```python
from build123d import *

# Parameters (mm, degrees)
SKETCH_1_R          = 17
EXTRUDE_1_DEPTH     = 6
SKETCH_2_R          = 7
EXTRUDE_2_DEPTH     = 6
SKETCH_3_R          = 18
EXTRUDE_3_DEPTH     = 5
EXTRUDE_START       = -5
EXTRUDE_6_DEPTH     = 5
CUT_EXTRUDE_1_DEPTH = 8
SKETCH_6_R          = 3.275
EXTRUDE_5_DEPTH     = 4.4
SKETCH_9_R          = 5
CUT_EXTRUDE_3_DEPTH = 37.608729958
SKETCH_10_R         = 13.6
SKETCH_10_R_2       = 8.6
CUT_EXTRUDE_4_DEPTH = 3


with BuildPart() as part:
    # 스케치1 → 보스-돌출1 (new body)
    with BuildSketch(Plane.XY):
        Circle(SKETCH_1_R)
    extrude(amount=EXTRUDE_1_DEPTH)

    # 스케치2 → 보스-돌출2 (add)
    with BuildSketch(Plane.XY.offset(6)):
        Circle(SKETCH_2_R)
    extrude(amount=EXTRUDE_2_DEPTH)

    # 스케치3 → 보스-돌출3 (add)
    with BuildSketch(Plane(origin=(0, 0, 0), x_dir=(-1, 0, 0), z_dir=(0, 0, -1))):
        Circle(SKETCH_3_R)
    extrude(amount=EXTRUDE_3_DEPTH)

    # 스케치8 → 보스-돌출6 (add)
    with BuildSketch(Plane(origin=(0, 0, -5), x_dir=(-1, 0, 0), z_dir=(0, 0, -1)).offset(EXTRUDE_START)):
        with BuildLine():
            Line((-10, 14.966629547), (-10, 26.966629547))
            Line((-10, 26.966629547), (10, 26.966629547))
            Line((10, 26.966629547), (10, 14.966629547))
            ThreePointArc((10, 14.966629547), (0, 18), (-10, 14.966629547))
        make_face()
    extrude_6 = extrude(amount=EXTRUDE_6_DEPTH)

    # 스케치5 → 컷-돌출1 (cut)
    with BuildSketch(Plane.XY):
        Polygon((-10, 27), (-10, 15), (-4, 27), align=None)
        Polygon((4, 27), (10, 27), (10, 15), align=None)
    cut_extrude_1 = extrude(amount=-CUT_EXTRUDE_1_DEPTH, mode=Mode.SUBTRACT)

    # 스케치6 → 보스-돌출5 (add)
    with BuildSketch(Plane.XY):
        with Locations(Location((0, 21.966629547, 0), (0, 0, 180))):
            Circle(SKETCH_6_R)
    extrude_5 = extrude(amount=EXTRUDE_5_DEPTH)

    # 대칭 복사6: 보스-돌출6, 컷-돌출1, 보스-돌출5 across plane
    add(extrude_6.mirror(Plane.ZX))
    add(cut_extrude_1.mirror(Plane.ZX), mode=Mode.SUBTRACT)
    add(extrude_5.mirror(Plane.ZX))

    # 스케치9 → 컷-돌출3 (cut, through all)
    with BuildSketch(Plane.XY.offset(12)):
        Circle(SKETCH_9_R)
    extrude(amount=-CUT_EXTRUDE_3_DEPTH, mode=Mode.SUBTRACT)

    # 스케치10 → 컷-돌출4 (cut)
    with BuildSketch(Plane(origin=(0, 0, -5), x_dir=(-1, 0, 0), z_dir=(0, 0, -1))):
        Circle(SKETCH_10_R)
        Circle(SKETCH_10_R_2, mode=Mode.SUBTRACT)
    extrude(amount=-CUT_EXTRUDE_4_DEPTH, mode=Mode.SUBTRACT)


solid = part.part
```
The model under review builds one solid part; all positions refer to its coordinate system, in mm. A direction names the side the tool comes from. Round coordinates to 2 decimals unless told otherwise and drop trailing zeros. Loops run counter-clockwise (first coordinate to the right, second up) from the corner with the lowest first, then second, coordinate; pieces in that order, holes last. Notation, with made-up numbers: (18, 73) -> (60, 73) arc R34 ccw to (60, 108) -> close; hole circle Ø5 at (39, 84). An arc over 180 degrees is marked (long way). Answer in a Markdown table with one row per item.
1) Wall thickness on line 1 along Y through (x, z) = (0, -3.3); line 2 along X through (y, z) = (2.5, -3.5); line 3 along X through (y, z) = (2.5, -1.25): over which ranges is each line inside the solid? List them lowest first.
Taken from the geometry:
| item | result |
|---|---|
| line 1 | y = -26.97 to -13.6, -8.6 to -5, 5 to 8.6, 13.6 to 26.97 |
| line 2 | x = -17.83 to -13.37, -8.23 to -4.33, 4.33 to 8.23, 13.37 to 17.83 |
| line 3 | x = -17.83 to -4.33, 4.33 to 17.83 |
2) Draft analysis for pull direction X (two halves, no side actions). For faces 5 (the cylindrical face through (-18, 0, -2)), 6 (the flat face through (12.3, 6.4, -5)), 7 (the cylindrical face through (9.139, 14.334, 2.958)), 8 (the cylindrical face through (2.948, -13.277, -3.521)), state which applies: pulls with the +X half, pulls with the -X half, needs draft (parallel to the pull), parting line crosses it, or undercut.
Taken from the geometry:
| item | result |
|---|---|
| face 5 | pulls with the -X half |
| face 6 | needs draft |
| face 7 | parting line crosses it |
| face 8 | undercut |
3) Tool access review of faces 1 (the flat face through (0, -9, -2)), 2 (the cylindrical face through (6.466, -2.681, 8.958)), 3 (the flat face through (0, -22, 4.4)), 4 (the flat face through (0, 22, 4.4)): name each direction out of +Z, -Z, +X, -X, +Y, -Y from which nothing blocks a thin tool from reaching the whole face with its end or side.
Taken from the geometry:
| item | result |
|---|---|
| face 1 | -Z |
| face 2 | +Z |
| face 3 | +Z, +X, -X, -Y |
| face 4 | +Z, +X, -X, +Y |
4) Consider section D-D, the plane x = 15. Write out the cut boundary in (y, z), plus the area to 3 significant figures.
Taken from the geometry:
| item | result |
|---|---|
| outline | (-9.95, -5) -> (9.95, -5) -> (9.95, 0) -> (8, 0) -> (8, 6) -> (-8, 6) -> (-8, 0) -> (-9.95, 0) -> close |
| area | 195 mm² |
5) Consider section C-C, the plane z = 10.25. Write out the cut boundary in (x, y).
Taken from the geometry:
| item | result |
|---|---|
| outline | circle Ø14 at (0, 0); hole circle Ø10 at (0, 0) |
6) Consider section B-B, the plane y = 2. Write out the cut boundary in (x, z).
Taken from the geometry:
| item | result |
|---|---|
| outline | (-17.89, -5) -> (-13.45, -5) -> (-13.45, -2) -> (-8.36, -2) -> (-8.36, -5) -> (-4.58, -5) -> (-4.58, 12) -> (-6.71, 12) -> (-6.71, 6) -> (-16.88, 6) -> (-16.88, 0) -> (-17.89, 0) -> close; (4.58, -5) -> (8.36, -5) -> (8.36, -2) -> (13.45, -2) -> (13.45, -5) -> (17.89, -5) -> (17.89, 0) -> (16.88, 0) -> (16.88, 6) -> (6.71, 6) -> (6.71, 12) -> (4.58, 12) -> close |
7) For pin 1 Ø17 at (x, y) = (0, -4.5) entering from +Z; pin 2 Ø5 at (x, y) = (-0.5, -22.5) entering from +Z; pin 3 Ø3 at (x, z) = (7.5, 3) entering from -Y; pin 4 Ø6 at (x, z) = (4, 3.5) entering from +Y, all flat-tipped, find the tip position at first contact; note any pin that passes through.
Taken from the geometry:
| item | result |
|---|---|
| pin 1 | stops at z = 12 |
| pin 2 | stops at z = 4.4 |
| pin 3 | stops at y = -15.91 |
| pin 4 | stops at y = 25.09 |
